Build history of the part. All positions in model axes, mm. Face numbers are marked on the shaded views. Round coordinates to 2 decimals unless told otherwise and drop trailing zeros. Order: outer loops, then holes, each group sorted by start corner. A loop starts at its lowest first (then second) coordinate and runs counter-clockwise, first axis right, second up. Notation, with made-up numbers: M 1.25,69.25 L 44.25,69.25 A22 cw 44.25,104.25 Z; hole C -1.75,11.25 d1. An arc over 180 degrees is marked long. One line per item, written item: value. Start each with the question number.
Item 1: Two-plate mould, pull along Z, no slides. Class the marked faces 1, 2, 3 and 4: +Z half, -Z half, draft (parallel to the pull), parting line (faces both ways), or undercut.
Item 2: Band-saw the part on D-D, the plane z = 20.25. Write the cut outline in (x, y), then the cut area to 3 significant figures.
Item 3: Probe L1, parallel to Y at x = 39.2, z = 27.25; L2, parallel to Z at x = 39.85, y = 19; L3, parallel to Y at x = 36.7, z = 23. List the from-to ranges inside material, lowest first.
Item 4: Band-saw the part on B-B, the plane z = 23. Write the cut outline in (x, y).
Item 5: Band-saw the part on C-C, the plane x = 38.25. Write the cut outline in (y, z), then the cut area to 3 significant figures.
Item 6: Pin check, flat tip, straight feed: pin 1 (2 mm diameter, centred on x = 38, z = 18, fed in from -Y). Stop position of the tip, or through.
Item 7: Band-saw the part on A-A, the plane y = 19. Write the cut outline in (x, z).
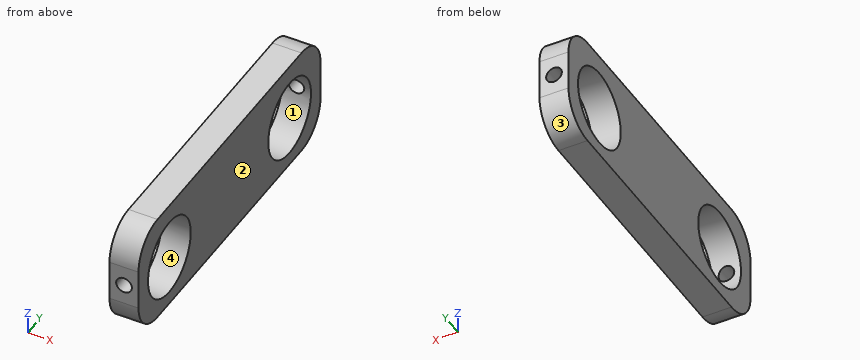
```python
from build123d import *

# Parameters (mm, degrees)
CYLINDER022_R     = 1.35
CYLINDER022_DEPTH = 10
CYLINDER021_R     = 1.35
CYLINDER021_DEPTH = 10
CYLINDER020_R     = 6.75
CYLINDER020_DEPTH = 50
CYLINDER019_R     = 6.75
CYLINDER019_DEPTH = 50
BOX005_W          = 5
BOX005_H          = 57.5
BOX005_DEPTH      = 19
FILLET007_R       = 6


with BuildPart() as cylinder017:
    # Cylinder022 → Cylinder022 (new body)
    with BuildSketch(Plane(origin=(2.5, -22, 23), x_dir=(1, 0, 0), z_dir=(0, -1, 0))):
        Circle(CYLINDER022_R)
    extrude(amount=CYLINDER022_DEPTH)


with BuildPart() as cylinder016:
    # Cylinder021 → Cylinder021 (new body)
    with BuildSketch(Plane(origin=(2.5, 32, 23), x_dir=(1, 0, 0), z_dir=(0, -1, 0))):
        Circle(CYLINDER021_R)
    extrude(amount=CYLINDER021_DEPTH)


with BuildPart() as tubo004:
    # Cylinder020 → Cylinder020 (new body)
    with BuildSketch(Plane(origin=(-24, 19, 22.5), x_dir=(0, 0, -1), z_dir=(1, 0, 0))):
        Circle(CYLINDER020_R)
    extrude(amount=CYLINDER020_DEPTH)


with BuildPart() as tubo003:
    # Cylinder019 → Cylinder019 (new body)
    with BuildSketch(Plane(origin=(-24, -19, 22.5), x_dir=(0, 0, -1), z_dir=(1, 0, 0))):
        Circle(CYLINDER019_R)
    extrude(amount=CYLINDER019_DEPTH)


with BuildPart() as obj1:
    # Box005 → Box005 (new body)
    with BuildSketch(Plane(origin=(0, -28.75, 13.5), x_dir=(1, 0, 0), z_dir=(0, 0, 1))):
        with Locations((2.5, 28.75)):
            Rectangle(BOX005_W, BOX005_H)
    extrude(amount=BOX005_DEPTH)

    # Fillet007
    fillet007_edges = [obj1.edges().sort_by_distance(p)[0] for p in [
        (2.5, -28.75, 13.5),
        (2.5, -28.75, 32.5),
        (2.5, 28.75, 13.5),
        (2.5, 28.75, 32.5),
    ]]
    fillet(fillet007_edges, radius=FILLET007_R)

    # Cut016: cut tubo003
    add(tubo003.part, mode=Mode.SUBTRACT)

    # Cut017: cut tubo004
    add(tubo004.part, mode=Mode.SUBTRACT)

    # Cut018: cut Cylinder016
    add(cylinder016.part, mode=Mode.SUBTRACT)

    # Cut019: cut Cylinder017
    add(cylinder017.part, mode=Mode.SUBTRACT)


with BuildPart() as obj1_1:
    # Cut019 placement: moved
    add(obj1.part.moved(Location((36, 0, 0))))


solid = obj1_1.part
```
Output:
1. face 1: undercut
1. face 2: draft
1. face 3: -Z half
1. face 4: undercut
2. outline: M 36,-28.75 L 41,-28.75 L 41,-25.36 L 36,-25.36 Z; M 36,-12.64 L 41,-12.64 L 41,12.64 L 36,12.64 Z; M 36,25.36 L 41,25.36 L 41,28.75 L 36,28.75 Z
2. area: 160 mm²
3. L1: y = -28.7 to -23.8, -14.2 to 14.2, 23.8 to 28.7
3. L2: z = 13.5 to 15.75, 29.25 to 32.5
3. L3: y = -28.75 to -25.73, -12.27 to 12.27, 25.73 to 28.75
4. outline: M 36,-28.75 L 37.15,-28.75 L 37.15,-25.73 L 36,-25.73 Z; M 36,-12.27 L 41,-12.27 L 41,12.27 L 36,12.27 Z; M 36,25.73 L 37.15,25.73 L 37.15,28.75 L 36,28.75 Z; M 39.85,-28.75 L 41,-28.75 L 41,-25.73 L 39.85,-25.73 Z; M 39.85,25.73 L 41,25.73 L 41,28.75 L 39.85,28.75 Z
5. outline: M -28.75,19.5 A6 ccw -22.75,13.5 L 22.75,13.5 A6 ccw 28.75,19.5 L 28.75,21.67 L 25.7,21.67 A6.75 cw long 25.5,24.33 L 28.75,24.33 L 28.75,26.5 A6 ccw 22.75,32.5 L -22.75,32.5 A6 ccw -28.75,26.5 L -28.75,24.33 L -25.5,24.33 A6.75 cw long -25.7,21.67 L -28.75,21.67 Z
5. area: 759 mm²
6. pin 1: stops at y = -28.73
7. outline: M 36,13.5 L 41,13.5 L 41,15.75 L 36,15.75 Z; M 36,29.25 L 41,29.25 L 41,32.5 L 36,32.5 Z
